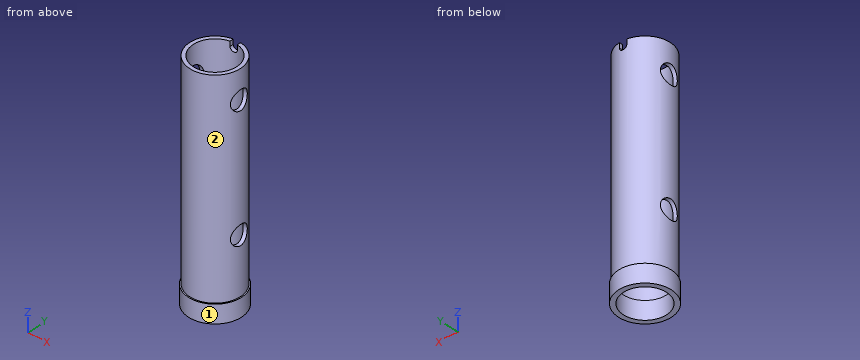
from build123d import *

# Parameters (mm, degrees)
SKETCH_1_R               = 11
SKETCH_1_R_2             = 9
EXTRUDE_1_DEPTH          = 7.5
SKETCH_3_R               = 10.5
SKETCH_3_R_2             = 9
EXTRUDE_2_DEPTH          = 86.25
CUT_EXTRUDE_1_DEPTH      = 86.25
CUT_EXTRUDE_1_DEPTH_BACK = 86.25
SKETCH_4_R               = 4
CUT_EXTRUDE_2_DEPTH      = 35.25


with BuildPart() as part:
    # 草图1 → 凸台-拉伸1 (new body)
    with BuildSketch(Plane.XY):
        with Locations(Location((-4.935418671, -158.561383044, 0), (0, 0, 180))):
            Circle(SKETCH_1_R)
        with Locations(Location((-4.935418671, -158.561383044, 0), (0, 0, 180))):
            Circle(SKETCH_1_R_2, mode=Mode.SUBTRACT)
    extrude(amount=EXTRUDE_1_DEPTH)

    # 草图3 → 凸台-拉伸2 (add)
    with BuildSketch(Plane.XY.offset(7.5)):
        with Locations(Location((-4.935418671, -158.561383044, 0), (0, 0, 180))):
            Circle(SKETCH_3_R)
        with Locations((-4.935418671, -158.561383044)):
            Circle(SKETCH_3_R_2, mode=Mode.SUBTRACT)
    extrude(amount=EXTRUDE_2_DEPTH)

    # 草图4 → 切除-拉伸1 (cut, two sides: drawn at the far end of the back side and taken through both)
    with BuildSketch(Plane(origin=(-8.503036589, -0.191549015, 0), x_dir=(0, 0, -1), z_dir=(0.9997463607277357, 0.022521416732707692, -5.695444116327053e-14)).offset(-CUT_EXTRUDE_1_DEPTH_BACK)):
        with Locations(Location((-81.75, -158.41001303, 0), (0, 0, 270))):
            Circle(SKETCH_4_R)
        with Locations(Location((-30.75, -158.41001303, 0), (0, 0, 270))):
            Circle(SKETCH_4_R)
    extrude(amount=CUT_EXTRUDE_1_DEPTH + CUT_EXTRUDE_1_DEPTH_BACK, mode=Mode.SUBTRACT)

    # 草图5 → 切除-拉伸2 (cut)
    with BuildSketch(Plane(origin=(3.567617918, -158.369834029, 0), x_dir=(0.9997463607277357, 0.022521416732707685, 0), z_dir=(-0.022521416732707685, 0.9997463607277357, 0))):
        with BuildLine():
            Line((-10.00519384, -93.75), (-10.00519384, -91.75))
            ThreePointArc((-10.00519384, -91.75), (-8.50519384, -90.25), (-7.00519384, -91.75))
            Line((-7.00519384, -91.75), (-7.00519384, -93.75))
            ThreePointArc((-7.00519384, -93.75), (-8.50519384, -95.25), (-10.00519384, -93.75))
        make_face()
    extrude(amount=CUT_EXTRUDE_2_DEPTH, mode=Mode.SUBTRACT)


solid = part.part
The listing builds one solid part. Answer for the finished solid, in the listing's coordinates (mm). Face numbers are marked on the shaded views. A direction names the side the tool comes from. Round coordinates to 2 decimals unless told otherwise and drop trailing zeros. Write each loop counter-clockwise with the first axis right and the second up, starting at its lowest first coordinate (ties: lowest second). Pieces come first, ordered by that corner, then holes. Notation, with made-up numbers: M 88.5,51 L 105.5,51 A31 ccw 105.5,81 Z; hole C 11,37 d4. An arc over 180 degrees is marked long. Write each question's results on one line, items separated by ' | '. Start each with the question number.
Item 1: A cutting plane is placed at D-D on y = -160.75. State how many separate pieces and enclosed holes the cut face has, and give its area (3 significant figures).
Item 2: Flat-ended cylindrical pins translate along their axes: pin 1 Ø2 at (y, z) = (-153.5, 14.5) entering from +X; pin 2 Ø10 at (x, z) = (-11.5, 49.5) entering from +Y; pin 3 Ø8 at (y, z) = (-161, 65.5) entering from +X. Find the tip coordinate at first contact, or state that the pin passes through.
Item 3: A cutting plane is placed at A-A on x = 1.75. Write down the section's boundary in (y, z).
Item 4: For the marked faces 1 and 2, determine the directions among +Z, -Z, +X, -X, +Y, -Y from which every point of the face is accessible in a straight line to the end or side of a thin tool.
Item 5: A cutting plane is placed at B-B on y = -165.25. Write down the section's boundary in (x, z).
Item 6: Straight lines are drawn through the part: L1, parallel to X at y = -158.5, z = 49; L2, parallel to X at y = -166, z = 25.5; L3, parallel to Z at x = -0.5, y = -168.25. For each, find the intervals that lie inside material, in ascending order. Write a range as [from, to].
Item 7: A cutting plane is placed at C-C on z = 14.5. Write down the section's boundary in (x, y).
Check sheet entries:
1) separate pieces: 6 | enclosed holes: 0 | area: 255 mm²
2) pin 1: x = 4.75 | pin 2: y = -148.18 | pin 3: x = 5.56
3) outline: M -167.3,0 L -164.59,0 L -164.59,93.75 L -166.66,93.75 L -166.66,7.5 L -167.3,7.5 Z; M -152.54,0 L -149.83,0 L -149.83,7.5 L -150.46,7.5 L -150.46,93.75 L -152.54,93.75 Z
4) face 1: +Z, -Z | face 2: +Z
5) outline: M -13.67,0 L -10.96,0 L -10.96,93.75 L -13.03,93.75 L -13.03,7.5 L -13.67,7.5 Z; M 1.09,0 L 3.8,0 L 3.8,7.5 L 3.16,7.5 L 3.16,93.75 L 1.09,93.75 Z
6) L1: [-15.44, -13.94], [4.06, 5.56] | L2: [-12.35, -10], [0.13, 2.48] | L3: [0, 7.5]
7) outline: C -4.94,-158.56 d21; hole C -4.94,-158.56 d18
